```python
from build123d import *

# Parameters (mm, degrees)
SKETCH_1_R      = 2
SKETCH_1_R_2    = 1.5
EXTRUDE_1_DEPTH = 5


with BuildPart() as part:
    # 草图1 → 凸台-拉伸1 (new body)
    with BuildSketch(Plane(origin=(0, 0, 0), x_dir=(1, 0, 0), z_dir=(0, 1, 0))):
        with BuildLine():
            Line((0, 12.5), (30, 12.5))
            ThreePointArc((30, 12.5), (42.5, 0), (30, -12.5))
            Line((30, -12.5), (0, -12.5))
            ThreePointArc((0, -12.5), (-12.5, 0), (0, 12.5))
        make_face()
        with Locations(Location((30, 0, 0), (0, 0, 270))):
            Circle(SKETCH_1_R, mode=Mode.SUBTRACT)
        with Locations(Location((0, 0, 0), (0, 0, 270))):
            Circle(SKETCH_1_R, mode=Mode.SUBTRACT)
        with Locations(Location((7, 0, 0), (0, 0, 270))):
            Circle(SKETCH_1_R_2, mode=Mode.SUBTRACT)
        with Locations(Location((0, 7, 0), (0, 0, 270))):
            Circle(SKETCH_1_R_2, mode=Mode.SUBTRACT)
        with Locations(Location((-7, 0, 0), (0, 0, 270))):
            Circle(SKETCH_1_R_2, mode=Mode.SUBTRACT)
        with Locations(Location((0, -7, 0), (0, 0, 270))):
            Circle(SKETCH_1_R_2, mode=Mode.SUBTRACT)
        with Locations(Location((23, 0, 0), (0, 0, 90))):
            Circle(SKETCH_1_R_2, mode=Mode.SUBTRACT)
        with Locations(Location((30, -7, 0), (0, 0, 90))):
            Circle(SKETCH_1_R_2, mode=Mode.SUBTRACT)
        with Locations(Location((37, 0, 0), (0, 0, 90))):
            Circle(SKETCH_1_R_2, mode=Mode.SUBTRACT)
        with Locations(Location((30, 7, 0), (0, 0, 90))):
            Circle(SKETCH_1_R_2, mode=Mode.SUBTRACT)
    extrude(amount=EXTRUDE_1_DEPTH)


solid = part.part
```
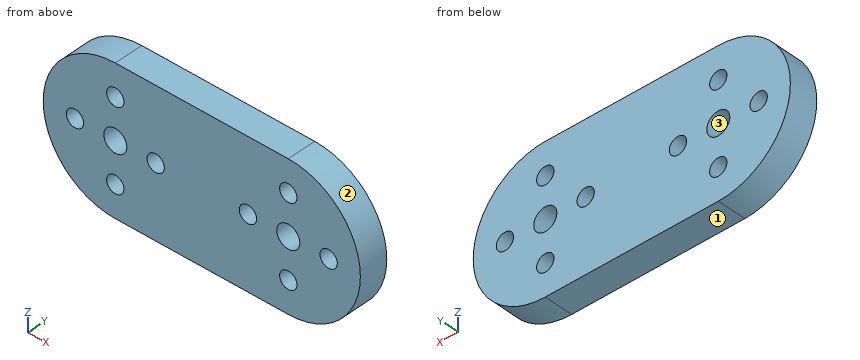
Can you work these out from the model? Positions are in its coordinate system, mm. Face numbers are marked on the shaded views. Round coordinates to 2 decimals unless told otherwise and drop trailing zeros. Loops run counter-clockwise (first coordinate to the right, second up) from the corner with the lowest first, then second, coordinate; pieces in that order, holes last. Notation, with made-up numbers: M -35.75,-22.5 L -16.75,-22.5 A13 ccw -16.75,-8.5 Z; hole C -21,45.5 d8. An arc over 180 degrees is marked long. Answer as a JSON object with one key per item and string values. Group by question number.
Q1. Imagine slicing it at C-C, the plane z = -0.25. Please give me the cut outline in (x, y), then the cut area to 3 significant figures.
Q2. Imagine slicing it at A-A, the plane y = 1.6. Count the separate pieces of the cut face and the enclosed holes in it, then the cut area to 3 significant figures.
Q3. Imagine slicing it at D-D, the plane x = -7. Please give me the cut outline in (y, z), then the cut area to 3 significant figures.
Q4. Will these pins go through, and if not, where does the flat tip stop? pin 1 (1.8 mm diameter, centred on x = 0, z = 7, fed in from -Y); pin 2 (1 mm diameter, centred on y = 2.5, z = -7, fed in from +X).
Q5. We'd pull the mould along X, two halves only. Please class the marked faces 1, 2 and 3: +X half, -X half, draft (parallel to the pull), parting line (faces both ways), or undercut.
Q6. Please list where these lines run through material, in increasing order: L1, parallel to X at y = 4.3, z = 1.75; L2, parallel to Z at x = 29.5, y = 2.2; L3, parallel to X at y = 2.45, z = -7.
Q7. Imagine slicing it at B-B, the plane x = 7. Please give me the cut outline in (y, z).
Findings:
{
 "1": {"outline": "M -12.5,0 L -8.48,0 L -8.48,5 L -12.5,5 Z; M -5.52,0 L -1.98,0 L -1.98,5 L -5.52,5 Z; M 1.98,0 L 5.52,0 L 5.52,5 L 1.98,5 Z; M 8.48,0 L 21.52,0 L 21.52,5 L 8.48,5 Z; M 24.48,0 L 28.02,0 L 28.02,5 L 24.48,5 Z; M 31.98,0 L 35.52,0 L 35.52,5 L 31.98,5 Z; M 38.48,0 L 42.5,0 L 42.5,5 L 38.48,5 Z", "area": "176 mm2"},
 "2": {"separate pieces": "1", "enclosed holes": "10", "area": "1,160 mm2"},
 "3": {"outline": "M 0,-10.36 L 5,-10.36 L 5,-1.5 L 0,-1.5 Z; M 0,1.5 L 5,1.5 L 5,10.36 L 0,10.36 Z", "area": "88.6 mm2"},
 "4": {"pin 1": "passes through", "pin 2": "stops at x = 40.68"},
 "5": {"face 1": "draft", "face 2": "+X half", "face 3": "undercut"},
 "6": {"L1": "x = -12.38 to -0.97, 0.97 to 29.03, 30.97 to 42.38", "L2": "z = -12.5 to -8.41, -5.59 to -1.94, 1.94 to 5.59, 8.41 to 12.5", "L3": "x = -10.36 to -1.5, 1.5 to 28.5, 31.5 to 40.36"},
 "7": {"outline": "M 0,-12.5 L 5,-12.5 L 5,-1.5 L 0,-1.5 Z; M 0,1.5 L 5,1.5 L 5,12.5 L 0,12.5 Z"}
}
